Work out the finished part from the listing and answer in its coordinate system (mm). A direction names the side the tool comes from. Coordinates: 2 decimals unless noted, no trailing zeros. Loops run counter-clockwise (first coordinate to the right, second up) from the corner with the lowest first, then second, coordinate; pieces in that order, holes last. Notation, with made-up numbers: (37, 71.5) - (87, 71.5) arc R23 ccw to (87, 102.5) - close; hole circle Ø2 at (59, -13). An arc over 180 degrees is marked (long way). Write each question's results on one line, items separated by ' | '. Start each with the question number.
Item 1: Each of these flat-tipped pins is pushed along its axis until it touches: pin 1 Ø7 at (y, z) = (45, 45) entering from +X; pin 2 Ø10 at (x, y) = (28, 24.5) entering from +Z; pin 3 Ø6 at (x, y) = (5, 10.5) entering from +Z; pin 4 Ø12 at (y, z) = (24, 24) entering from +X. Where does it stop, or does it pass through?
Item 2: Section D-D, the plane y = 46 is taken. Write down the section's boundary in (x, z).
Item 3: Consider probe 1 along Y at (x, z) = (74, 45); probe 2 along Z at (x, y) = (41.5, 24.5); probe 3 along X at (y, z) = (32.5, 4). Determine where each line is inside the solid, lowest interval first. Write a range as [from, to].
Item 4: Section B-B, the plane y = 25 is taken. Write down the section's boundary in (x, z).
Item 5: For a pull along Y with two mould halves and no side action, classify faces 1 (the face through (75.07, 47.03, 47.21)), 2 (the face through (75, 50, 25)), 3 (the face through (75, 1, 2)), 4 (the face through (-5, 25, 50)) as +Y half, -Y half, draft (parallel to the pull), parting line (faces both ways), or undercut.
Item 6: Section C-C, the plane x = -3 is taken. Write down the section's boundary in (y, z).
Item 7: Section A-A, the plane x = 24 is taken. Write down the section's boundary in (y, z).
Item 8: A tool of negligible diameter and unlimited length cuts with its end or side. For faces 5 (the face through (70, 25, 48)), 6 (the face through (35, 25, 5)), 7 (the face through (35.49, 7.85, 8.01)), 8 (the face through (35, 25, 45)), from which of +Z, -Z, +X, -X, +Y, -Y can it reach the whole face along a straight path? Write none if from no direction.
Autodesk Inventor part; units mm, degrees
ref_plane "YZ Plane" through (0, 0, 0) normal (1, 0, 0) x (0, 1, 0)
ref_plane "XZ Plane" through (0, 0, 0) normal (0, 1, 0) x (-1, 0, 0)
ref_plane "XY Plane" through (0, 0, 0) normal (0, 0, 1) x (1, 0, 0)
sketch "Sketch1" plane through (0, 0, 0) normal (1, 0, 0) x (0, 1, 0)
  line L0 (0, 0) -> (50, 0)
  line L1 (50, 0) -> (50, 50)
  line L2 (50, 50) -> (0, 50)
  line L3 (0, 50) -> (0, 0)
  circle A0 centre (25, 25) radius 7.5
  dimension "d0" = 50
  dimension "d1" = 50
  dimension "d2" = 15
extrude "Extrusion1" add sketch "Sketch1" along normal blind 80
extrude "Extrusion2" add sketch "Sketch1" against normal blind 10 contours L3 L2 L1 L0 | A0
sketch "Sketch2" plane through (80, 0, 50) normal (0, 0, 1) x (1, 0, 0)
  line L0 (0, 50) -> (-90, 50)
  line L1 (-90, 0) -> (0, 0)
  line L2 (-80, 50) -> (-10, 50)
  line L3 (-10, 50) -> (-10, 0)
  line L4 (-10, 0) -> (-80, 0)
  line L5 (-80, 0) -> (-80, 50)
  line L6 (-80, 50) -> (-10, 50)
  line L7 (-10, 50) -> (-10, 45)
  line L8 (-10, 45) -> (-80, 45)
  line L9 (-80, 45) -> (-80, 50)
  line L10 (-10, 0) -> (-80, 0)
  line L11 (-80, 0) -> (-80, 5)
  line L12 (-80, 5) -> (-10, 5)
  line L13 (-10, 5) -> (-10, 0)
  point P0 (-10, 45)
  dimension "d7" = 70
  dimension "d8" = 70
  dimension "d9" = 5
  dimension "d10" = 70
  dimension "d11" = 5
extrude "Extrusion3" cut sketch "Sketch2" against normal blind 50 contours L3 L8 L5 L0 | L3 L1 L5 L12
extrude "Extrusion4" cut sketch "Sketch2" against normal blind 5 contours L3 L12 L5 L8
sketch "Sketch3" plane through (80, 0, 0) normal (0, 0, -1) x (-1, 0, 0)
  line L0 (80, 45) -> (10, 45)
  line L1 (80, 5) -> (80, 0)
  line L2 (10, 45) -> (80, 45)
  line L3 (80, 45) -> (80, 5)
  line L4 (80, 5) -> (10, 5)
  line L5 (10, 5) -> (10, 45)
extrude "Extrusion5" cut sketch "Sketch3" against normal blind 5
fillet "Fillet2" radius 5 8 edges at (-5, 50, 50) (75, 50, 50) (75, 50, 0) (-5, 50, 0) (-5, 0, 0) (75, 0, 0) (-5, 0, 50) (75, 0, 50)
fillet "Fillet3" radius 10 4 edges at (35, 45, 45) (35, 5, 45) (35, 45, 5) (35, 5, 5)
sketch "Sketch5" plane through (80, 0, 0) normal (1, 0, 0) x (0, 0, -1)
  arc A0 (-45, 50) -> (-50, 45) centre (-45, 45) ccw
  circle A1 centre (-45, 45) radius 3
  arc A2 (0, 45) -> (-5, 50) centre (-5, 45) ccw
  circle A3 centre (-5, 45) radius 3
  arc A4 (-5, 0) -> (0, 5) centre (-5, 5) ccw
  circle A5 centre (-5, 5) radius 3
  arc A6 (-50, 5) -> (-45, 0) centre (-45, 5) ccw
  circle A7 centre (-45, 5) radius 3
  point P0 (0, 0)
  dimension "d25" = 6
  dimension "d26" = 6
  dimension "d27" = 6
  dimension "d28" = 6
extrude "Extrusion6" cut sketch "Sketch5" against normal blind 90
properties part number "Contenedor"
Answer key:
1) pin 1: stops at x = 80 | pin 2: stops at z = 45 | pin 3: stops at z = 44.89 | pin 4: stops at x = 0
2) outline: (-10, 0.1) - (0, 0.1) - (0, 2.17) - (-10, 2.17) - close; (-10, 7.83) - (0, 7.83) - (0, 42.17) - (-10, 42.17) - close; (-10, 47.83) - (0, 47.83) - (0, 49.9) - (-10, 49.9) - close; (70, 0.1) - (80, 0.1) - (80, 2.17) - (70, 2.17) - close; (70, 7.83) - (80, 7.83) - (80, 42.17) - (70, 42.17) - close; (70, 47.83) - (80, 47.83) - (80, 49.9) - (70, 49.9) - close
3) probe 1: y = [0, 2], [8, 42], [48, 50] | probe 2: z = [5, 17.52], [32.48, 45] | probe 3: x = [-10, 0], [70, 80]
4) outline: (-10, 0) - (0, 0) - (0, 5) - (70, 5) - (70, 0) - (80, 0) - (80, 17.5) - (0, 17.5) - (0, 32.5) - (80, 32.5) - (80, 50) - (70, 50) - (70, 45) - (0, 45) - (0, 50) - (-10, 50) - close
5) face 1: undercut | face 2: +Y half | face 3: -Y half | face 4: draft
6) outline: (0, 5) arc R5 ccw to (5, 0) - (45, 0) arc R5 ccw to (50, 5) - (50, 45) arc R5 ccw to (45, 50) - (5, 50) arc R5 ccw to (0, 45) - close; hole circle Ø6 at (5, 5); hole circle Ø6 at (5, 45); hole circle Ø6 at (45, 5); hole circle Ø6 at (45, 45)
7) outline: (5, 15) arc R10 ccw to (15, 5) - (35, 5) arc R10 ccw to (45, 15) - (45, 35) arc R10 ccw to (35, 45) - (15, 45) arc R10 ccw to (5, 35) - close; hole circle Ø15 at (25, 25)
8) face 5: none | face 6: -Z, +Y, -Y | face 7: -Z, -Y | face 8: +Z, +Y, -Y
